Geometry check sheet. Reference: the model listing, model coordinates, mm. Face numbers are marked on the shaded views. A direction names the side the tool comes from. Give positions to 0.01 mm unless a question says otherwise; leave off trailing zeros. Write each loop counter-clockwise with the first axis right and the second up, starting at its lowest first coordinate (ties: lowest second). Pieces come first, ordered by that corner, then holes. Notation, with made-up numbers: (-7, 5) -> (23, 5) arc R16 cw to (23, 11) -> close; hole circle Ø6 at (82, -30.5). An arc over 180 degrees is marked (long way). Write item = value, one per line. Start each with the question number.
1. Thickness scan on line 1 along X through (y, z) = (10.05, -1); line 2 along X through (y, z) = (11.25, -4); line 3 along Y through (x, z) = (10.5, 3.5). Record the ranges inside material, lowest first.
2. Set-up check for the marked faces 4, 5, 6, 7 and 8: record each of +Z, -Z, +X, -X, +Y, -Y from which the full face is reachable in a straight line by a thin tool's end or side.
3. Mould release check, pull along X, two halves, no side actions. Record for the marked faces 1, 2 and 3: pulls with the +X half, pulls with the -X half, needs draft (parallel to the pull), parting line crosses it, or undercut.
4. Depth check by flat-ended pin: P1, Ø1.5, axis at y = 6.5, z = -7.5, coming from the -X side; P2, Ø4.5, axis at x = 10.5, y = 10, coming from the +Z side (3 decimals); P3, Ø4, axis at x = 10, y = 9, coming from the -Z side (3 decimals). Enter the tip coordinate at first touch or a pass-through.
5. Cross-section at B-B, the plane x = 5.5. Record the cut outline in (y, z) (3 decimals), plus the area to 3 significant figures.
6. Cross-section at A-A, the plane z = 5.5. Record the cut outline in (x, y) (3 decimals).
```python
from build123d import *

# Parameters (mm, degrees)
BOSS_EXTRUDE1_DEPTH = 70
SKETCH2_R           = 2
CUT_EXTRUDE1_DEPTH  = 15
SKETCH3_R           = 2
CUT_EXTRUDE2_DEPTH  = 15
CUT_EXTRUDE3_START  = -3
CUT_EXTRUDE3_DEPTH  = 3
CUT_EXTRUDE4_START  = -3
CUT_EXTRUDE4_DEPTH  = 3
FILLET1_R           = 2
SKETCH8_W           = 45.954012469
SKETCH8_H           = 31.924176852
CUT_EXTRUDE6_DEPTH  = 53
CUT_EXTRUDE7_START  = -3
CUT_EXTRUDE7_DEPTH  = 3
CUT_EXTRUDE8_START  = -3
CUT_EXTRUDE8_DEPTH  = 3
SKETCH11_R          = 2.3876
CUT_EXTRUDE9_DEPTH  = 6.35
CUT_EXTRUDE9_DRAFT  = -8
SKETCH12_R          = 1.4951657
CUT_EXTRUDE10_DEPTH = 5
FILLET2_R           = 1


with BuildPart() as part:
    # Sketch1 → Boss-Extrude1 (new body)
    with BuildSketch(Plane(origin=(0, 0, 0), x_dir=(1, 0, 0), z_dir=(0, 1, 0))):
        with BuildLine():
            Line((-18.495, 5.34), (-9.495, 17.34))
            Line((-9.495, 17.34), (2.725, 8.175))
            Line((2.725, 8.175), (18, 8.175))
            Line((18, 8.175), (18, -6.825))
            Line((18, -6.825), (3, -6.825))
            Line((3, -6.825), (3, -10))
            Line((3, -10), (0, -10))
            ThreePointArc((0, -10), (-3.16227766, -9.486832981), (-6, -8))
            Line((-6, -8), (-8.4, -6.2))
            Line((-8.4, -6.2), (-6.495, -3.66))
            Line((-6.495, -3.66), (-18.495, 5.34))
        make_face()
    extrude(amount=BOSS_EXTRUDE1_DEPTH)

    # Sketch2 → Cut-Extrude1 (cut)
    with BuildSketch(Plane.XY.offset(6.825)):
        with Locations((10.5, 10)):
            Circle(SKETCH2_R)
        with Locations((10.5, 60)):
            Circle(SKETCH2_R)
    extrude(amount=-CUT_EXTRUDE1_DEPTH, mode=Mode.SUBTRACT)

    # Sketch3 → Cut-Extrude2 (cut)
    with BuildSketch(Plane(origin=(-4.095, 0, 5.46), x_dir=(0.8000000000000002, 0, 0.5999999999999999), z_dir=(-0.5999999999999999, 0, 0.8000000000000003))):
        with Locations((-10.5, 10)):
            Circle(SKETCH3_R)
        with Locations((-10.5, 60)):
            Circle(SKETCH3_R)
    extrude(amount=-CUT_EXTRUDE2_DEPTH, mode=Mode.SUBTRACT)

    # Sketch4 → Cut-Extrude3 (cut)
    with BuildSketch(Plane(origin=(4.905, 0, -6.54), x_dir=(-0.8000000000000002, 0, -0.5999999999999998), z_dir=(0.5999999999999998, 0, -0.8000000000000002)).offset(CUT_EXTRUDE3_START)):
        Polygon((6.28125, 12.435696448), (10.5, 14.871392896), (14.71875, 12.435696448), (14.71875, 0), (6.28125, 0), align=None)
        Polygon((10.5, 55.128607104), (14.71875, 57.564303552), (14.71875, 62.435696448), (10.5, 64.871392896), (6.28125, 62.435696448), (6.28125, 57.564303552), align=None)
    extrude(amount=-CUT_EXTRUDE3_DEPTH, mode=Mode.SUBTRACT)

    # Sketch5 → Cut-Extrude4 (cut)
    with BuildSketch(Plane(origin=(0, 0, -8.175), x_dir=(-1, 0, 0), z_dir=(0, 0, -1)).offset(CUT_EXTRUDE4_START)):
        Polygon((-14.71875, 12.435696448), (-10.5, 14.871392896), (-6.28125, 12.435696448), (-6.28125, 0), (-14.71875, 0), align=None)
        Polygon((-10.5, 55.128607104), (-6.28125, 57.564303552), (-6.28125, 62.435696448), (-10.5, 64.871392896), (-14.71875, 62.435696448), (-14.71875, 57.564303552), align=None)
    extrude(amount=-CUT_EXTRUDE4_DEPTH, mode=Mode.SUBTRACT)

    # Fillet1
    fillet1_edges = [part.edges().sort_by_distance(p)[0] for p in [
        (-13.995, 0, -11.34),
        (18, 0, -0.675),
        (-18.495, 35, -5.34),
        (-9.495, 35, -17.34),
        (2.725, 35, -8.175),
        (18, 35, -8.175),
        (18, 35, 6.825),
    ]]
    fillet(fillet1_edges, radius=FILLET1_R)

    # Sketch8 → Cut-Extrude6 (cut)
    with BuildSketch(Plane(origin=(0, 70, 0), x_dir=(1, 0, 0), z_dir=(0, 1, 0))):
        with Locations((-0.294273389, 3.101020579)):
            Rectangle(SKETCH8_W, SKETCH8_H)
    extrude(amount=-CUT_EXTRUDE6_DEPTH, mode=Mode.SUBTRACT)

    # Sketch9 → Cut-Extrude7 (cut)
    with BuildSketch(Plane(origin=(4.905, 0, -6.54), x_dir=(-0.8000000000000002, 0, -0.5999999999999998), z_dir=(0.5999999999999998, 0, -0.8000000000000002)).offset(CUT_EXTRUDE7_START)):
        with BuildLine():
            Line((12.5, 10), (12.5, 0))
            Line((12.5, 0), (8.5, 0))
            Line((8.5, 0), (8.5, 10))
            ThreePointArc((8.5, 10), (10.5, 8), (12.5, 10))
        make_face()
    extrude(amount=CUT_EXTRUDE7_DEPTH, mode=Mode.SUBTRACT)

    # Sketch10 → Cut-Extrude8 (cut)
    with BuildSketch(Plane(origin=(0, 0, -8.175), x_dir=(-1, 0, 0), z_dir=(0, 0, -1)).offset(CUT_EXTRUDE8_START)):
        with BuildLine():
            Line((-8.5, 10), (-8.5, 0))
            Line((-8.5, 0), (-12.5, 0))
            Line((-12.5, 0), (-12.5, 10))
            ThreePointArc((-12.5, 10), (-10.5, 8), (-8.5, 10))
        make_face()
    extrude(amount=CUT_EXTRUDE8_DEPTH, mode=Mode.SUBTRACT)


with BuildPart() as cut_extrude9_tool:
    # Sketch11 → Cut-Extrude9 (with draft: the straight prism first)
    with BuildSketch(Plane.XZ):
        with Locations((0.333333333, -1)):
            Circle(SKETCH11_R)
    extrude(amount=-CUT_EXTRUDE9_DEPTH)
    # Cut-Extrude9: the draft: its side faces are tilted about the plane it starts from
    cut_extrude9_sides = [cut_extrude9_tool.faces().sort_by_distance(p)[0] for p in [
        (-2.054266667, 3.175, -1),
    ]]
    draft(cut_extrude9_sides, Plane.XZ, CUT_EXTRUDE9_DRAFT)


with BuildPart() as part_1:
    add(part.part)

    # Cut-Extrude9: cut by cut_extrude9_tool
    add(cut_extrude9_tool.part, mode=Mode.SUBTRACT)

    # Sketch12 → Cut-Extrude10 (cut)
    with BuildSketch(Plane.XZ.offset(-6.35)):
        with Locations(Location((0.333333333, -1, 0), (0, 0, 270))):
            Circle(SKETCH12_R)
    extrude(amount=-CUT_EXTRUDE10_DEPTH, mode=Mode.SUBTRACT)

    # Fillet2
    fillet2_edges = [part_1.edges().sort_by_distance(p)[0] for p in [
        (-5.995, 0, -12.84),
        (-2.795, 0, -10.44),
        (8.5, 0, -6.675),
        (12.5, 0, -6.675),
    ]]
    fillet(fillet2_edges, radius=FILLET2_R)


solid = part_1.part
```
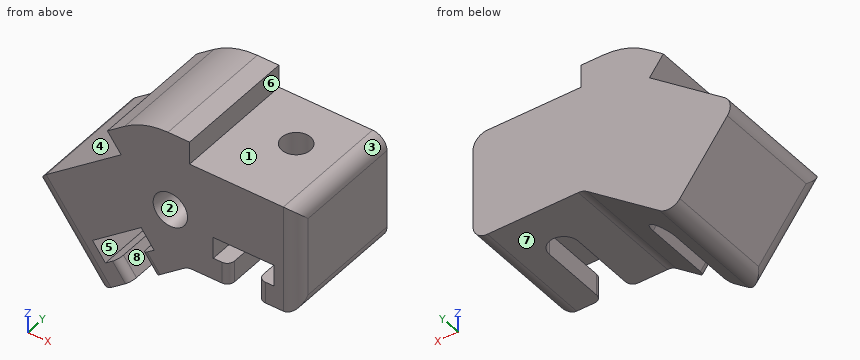
Answers:
q1.line_1 = -9.88 to -1.16, 1.83 to 8.5, 12.5 to 18
q1.line_2 = -16.71 to -12.08, -8.17 to 6.28, 14.72 to 18
q1.line_3 = 0 to 8, 12 to 17
q2.face_4 = -X, +Y, -Y
q2.face_5 = -Y
q2.face_6 = +Z, +X, +Y, -Y
q2.face_7 = -Z, +X, +Y, -Y
q2.face_8 = +X, -Y
q3.face_1 = needs draft
q3.face_2 = undercut
q3.face_3 = pulls with the +X half
q4.P1 = -17.42
q4.P2 = 6.825
q4.P3 = -8.175
q5.outline = (0, -8.175) -> (17, -8.175) -> (17, 6.825) -> (0, 6.825) -> close
q5.area = 255 mm^2
q6.outline = (-7.875, 0) -> (16, 0) arc R2 ccw to (17.883, 1.325) -> (17.883, 17) -> (-7.875, 17) -> close; hole circle Ø4 at (10.5, 10)
